Read the model definition and answer for the solid it produces. Units are mm, in the model's axes. Face numbers are marked on the shaded views. A direction names the side the tool comes from. Round coordinates to 2 decimals unless told otherwise and drop trailing zeros. Loops run counter-clockwise (first coordinate to the right, second up) from the corner with the lowest first, then second, coordinate; pieces in that order, holes last. Notation, with made-up numbers: M 22,53 L 77,53 A17 cw 77,63 Z; hole C 55,64.5 d8. An arc over 180 degrees is marked long. Answer as CSV lines item,"result".
```python
from build123d import *

# Parameters (mm, degrees)
SKETCH1_R                = 4.7625
BOSS_EXTRUDE1_DEPTH      = 12.7
BOSS_EXTRUDE2_DEPTH      = 6.35
BOSS_EXTRUDE2_DEPTH_BACK = 19.05
SKETCH4_W                = 20.078494948
SKETCH4_H                = 48.78095735
SKETCH4_W_2              = 48.420880553
SKETCH4_H_2              = 19.195923741
CUT_EXTRUDE2_DEPTH       = 26.162
SKETCH5_R                = 3.175
CUT_EXTRUDE3_DEPTH       = 11.43
SKETCH6_R                = 3.175
CUT_EXTRUDE4_DEPTH       = 11.43
SKETCH11_R               = 2
CUT_EXTRUDE7_DEPTH       = 21.844


with BuildPart() as part:
    # Sketch1 → Boss-Extrude1 (new body)
    with BuildSketch(Plane(origin=(0, 0, 0), x_dir=(0, 0, -1), z_dir=(1, 0, 0))):
        with BuildLine():
            Line((0, 31.882172919), (31.882172919, 31.882172919))
            Line((31.882172919, 31.882172919), (60.87463474, 31.882172919))
            Line((60.87463474, 31.882172919), (60.87463474, -60.96))
            Line((60.87463474, -60.96), (-31.882172919, -60.96))
            Line((-31.882172919, -60.96), (-31.882172919, 0))
            ThreePointArc((-31.882172919, 0), (-22.54410067, 22.54410067), (0, 31.882172919))
        make_face()
        Circle(SKETCH1_R, mode=Mode.SUBTRACT)
    extrude(amount=BOSS_EXTRUDE1_DEPTH)

    # Sketch8 → Boss-Extrude2 (add, two sides: drawn at the far end of the back side and taken through both)
    with BuildSketch(Plane(origin=(12.7, 0, 0), x_dir=(0, 0, -1), z_dir=(1, 0, 0)).offset(-BOSS_EXTRUDE2_DEPTH_BACK)):
        Polygon((60.87463474, 31.882172919), (53.770648903, 31.882172919), (53.770648903, -51.937867719), (-31.882172919, -51.937867719), (-31.882172919, -60.96), (53.770648903, -60.96), (60.87463474, -60.96), align=None)
    extrude(amount=BOSS_EXTRUDE2_DEPTH + BOSS_EXTRUDE2_DEPTH_BACK)

    # Sketch4 → Cut-Extrude2 (cut)
    with BuildSketch(Plane.ZY):
        with Locations((-43.731401429, -0.427222634)):
            Rectangle(SKETCH4_W, SKETCH4_H)
        with Locations((-0.75610861, -42.339905849)):
            Rectangle(SKETCH4_W_2, SKETCH4_H_2)
        with Locations((-43.731401429, -42.339905849)):
            Rectangle(SKETCH4_W, SKETCH4_H_2)
    extrude(amount=-CUT_EXTRUDE2_DEPTH, mode=Mode.SUBTRACT)

    # Sketch5 → Cut-Extrude3 (cut)
    with BuildSketch(Plane(origin=(0, 0, -60.87463474), x_dir=(-1, 0, 0), z_dir=(0, 0, -1))):
        with Locations((-6.35, 16.187024645)):
            Circle(SKETCH5_R)
        with Locations((-6.35, -44.788648077)):
            Circle(SKETCH5_R)
    extrude(amount=-CUT_EXTRUDE3_DEPTH, mode=Mode.SUBTRACT)

    # Sketch6 → Cut-Extrude4 (cut)
    with BuildSketch(Plane.XZ.offset(60.96)):
        with Locations(Location((6.35, 15.24, 0), (0, 0, 270))):
            Circle(SKETCH6_R)
        with Locations(Location((6.35, -45.41055385, 0), (0, 0, 270))):
            Circle(SKETCH6_R)
    extrude(amount=-CUT_EXTRUDE4_DEPTH, mode=Mode.SUBTRACT)

    # Sketch11 → Cut-Extrude7 (cut)
    with BuildSketch(Plane(origin=(12.7, 0, 0), x_dir=(0, 0, -1), z_dir=(1, 0, 0))):
        with Locations((7.5, 0)):
            Circle(SKETCH11_R)
        with Locations((0, -7.5)):
            Circle(SKETCH11_R)
        with Locations((-7.5, 0)):
            Circle(SKETCH11_R)
        with Locations((0, 7.5)):
            Circle(SKETCH11_R)
    extrude(amount=-CUT_EXTRUDE7_DEPTH, mode=Mode.SUBTRACT)


solid = part.part
```
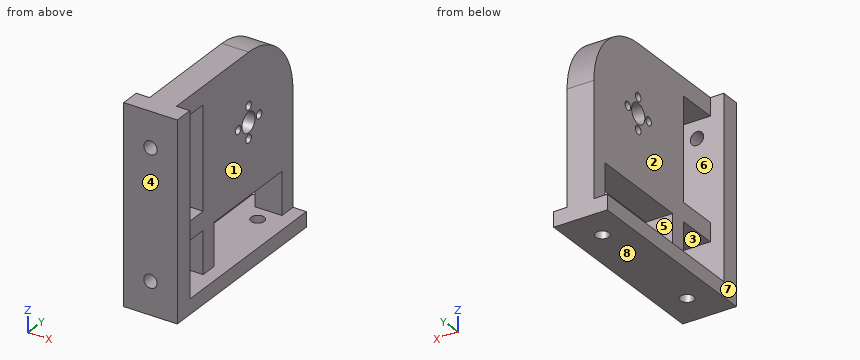
1) Find section C-C, the plane z = -15. Give the vertices of the cut face in (x, y).
Evaluation:
outline,"M -6.35,-60.96 L 19.05,-60.96 L 19.05,-51.94 L -6.35,-51.94 Z; M 0,-32.74 L 12.7,-32.74 L 12.7,31.88 L 0,31.88 Z"
2) Determine the mould class of the marked faces 5, 6, 7 and 8 for opening direction Z: released by +Z, released by -Z, zero draft, split by the parting line, or undercut.
Evaluation:
face 5,"undercut"
face 6,"undercut"
face 7,"zero draft"
face 8,"released by -Z"
3) Find section A-A, the plane z = -40. Give the vertices of the cut face in (x, y).
Evaluation:
outline,"M -6.35,-60.96 L 19.05,-60.96 L 19.05,-51.94 L -6.35,-51.94 Z; M 0,-32.74 L 12.7,-32.74 L 12.7,-24.82 L 0,-24.82 Z; M 0,23.96 L 12.7,23.96 L 12.7,31.88 L 0,31.88 Z"
4) A tool of negligible diameter and unlimited length cuts with its end or side. For the marked faces 1, 2, 3 and 4, from which of +Z, -Z, +X, -X, +Y, -Y can it reach the whole face along a straight path? Write none if from no direction.
Evaluation:
face 1,"+Z, +X, +Y"
face 2,"+Z, -X, +Y"
face 3,"+X, -X"
face 4,"+Z, -Z, +X, -X, -Y"
5) Find section B-B, the plane y = -7.5. Give the vertices of the cut face in (x, z), then the cut area to 3 significant figures.
Evaluation:
outline,"M -6.35,-60.87 L 19.05,-60.87 L 19.05,-53.77 L -6.35,-53.77 Z; M 0,-33.69 L 12.7,-33.69 L 12.7,-2 L 0,-2 Z; M 0,2 L 12.7,2 L 12.7,31.88 L 0,31.88 Z"
area,"962 mm^2"
6) Straight lines are drawn through the part: line 1 (Y direction, x = 6.75, z = -35.5); line 2 (Y direction, x = 6.35, z = -57.25); line 3 (Z direction, x = 6.25, y = -18). For each, find the intervals that lie inside material, in ascending order.
Evaluation:
line 1,"y = -60.96 to -51.94, -32.74 to -24.82, 23.96 to 31.88"
line 2,"y = -60.96 to -47.96, -41.61 to 13.01, 19.36 to 31.88"
line 3,"z = -60.87 to -53.77, -33.69 to 31.88"
7) Find section D-D, the plane x = 6.35. Count the separate pieces of the cut face and the enclosed holes in it, then the cut area to 3 significant figures.
Evaluation:
separate pieces,"2"
enclosed holes,"5"
area,"5,770 mm^2"
8) This flat-tipped pin is pushed along its axis until it touches: P1, Ø6, axis at y = -21, z = -9, coming from the +X side. Where does it stop, or does it pass through?
Evaluation:
P1,"stops at x = 12.7"
